Can you work these out from the model? Positions are in its coordinate system, mm. Face numbers are marked on the shaded views. Give positions to 0.01 mm unless a question says otherwise; leave off trailing zeros. Loops run counter-clockwise (first coordinate to the right, second up) from the corner with the lowest first, then second, coordinate; pieces in that order, holes last. Notation, with made-up numbers: (41.25, -31) -> (94.25, -31) arc R16 ccw to (94.25, -6) -> close; hole circle Ø5 at (-11.5, 66.5). An arc over 180 degrees is marked (long way). Return JSON: item names as keys, results as strings. Group by question number.
Q1. Suppose I cut it at B-B, the plane y = -1.9. Please give me the cut outline in (x, z) (3 decimals).
Q2. Thinking about a two-plate mould opening in Y: for the marked faces 1 and 2, which applies, pulls with the +Y half, pulls with the -Y half, needs draft (parallel to the pull), parting line crosses it, or undercut?
Q3. Suppose I cut it at C-C, the plane z = -34. Please give me the cut outline in (x, y).
Q4. Suppose I cut it at A-A, the plane z = -18.35. Please give me the cut outline in (x, y), and give its area (3 significant figures).
Q5. Suppose I cut it at D-D, the plane x = 14.5. Please give me the cut outline in (y, z) (3 decimals), and give its area (3 significant figures).
Q6. I need wall thicknesses on line 1 along X through (y, z) = (-1.85, -18.35); line 2 along X through (y, z) = (-1.05, -44.5); line 3 along X through (y, z) = (-0.75, -6.5). Which ranges of each line are inside material? Lowest first, please. Write a range as [from, to].
Q7. Will these pins go through, and if not, where does the flat tip stop? pin 1 (1.6 mm diameter, centred on x = 2, y = -1, fed in from -Z) (3 decimals); pin 2 (1 mm diameter, centred on y = -3, z = -37, fed in from +X); pin 3 (1.5 mm diameter, centred on x = 13, y = -2.5, fed in from +Z).
```python
from build123d import *

# Parameters (mm, degrees)
BASE_FLANGE1_START        = -3.2
BASE_FLANGE1_DEPTH        = 3.2
SKETCH8_R                 = 1.635
CUT_EXTRUDE1_DEPTH        = 3.2
F_4_CLEARANCE_HOLE1_D     = 3.2639
F_4_CLEARANCE_HOLE1_DEPTH = 3.2
F_4_CLEARANCE_HOLE1_TIP   = 0.980574487
CUT_EXTRUDE2_DEPTH        = 3.2


# Read off the part's stored shape, not the designer's step: Base-Flange1
with BuildPart() as part:
    # Base-Flange1 outline → Base-Flange1 (new body)
    with BuildSketch(Plane(origin=(0, 0, 0), x_dir=(1, 0, 0), z_dir=(0, 1, 0)).offset(BASE_FLANGE1_START)):
        with BuildLine():
            ThreePointArc((-29.358964924, 3.232453337), (-23.15, 7), (-16.941035076, 3.232453337))
            ThreePointArc((-16.941035076, 3.232453337), (-11.575, 1.808851774), (-6.208964924, 3.232453337))
            ThreePointArc((-6.208964924, 3.232453337), (0, 7), (6.208964924, 3.232453337))
            ThreePointArc((6.208964924, 3.232453337), (11.575, 1.808851774), (16.941035076, 3.232453337))
            ThreePointArc((16.941035076, 3.232453337), (23.15, 7), (29.358964924, 3.232453337))
            Line((29.358964924, 3.232453337), (29.358964924, 25.825))
            Line((29.358964924, 25.825), (-19.358964924, 25.825))
            Line((-19.358964924, 25.825), (-19.358964924, 48.325))
            Line((-19.358964924, 48.325), (-29.358964924, 48.325))
            Line((-29.358964924, 48.325), (-29.358964924, 3.232453337))
        make_face()
    extrude(amount=BASE_FLANGE1_DEPTH)

    # Sketch8 → Cut-Extrude1 (cut)
    with BuildSketch(Plane(origin=(0, 0, 0), x_dir=(1, 0, 0), z_dir=(0, 1, 0))):
        with Locations(Location((-24.358964924, 44.325, 0), (0, 0, 270))):
            Circle(SKETCH8_R)
        with Locations(Location((-24.358964924, 34.825, 0), (0, 0, 270))):
            Circle(SKETCH8_R)
    extrude(amount=-CUT_EXTRUDE1_DEPTH, mode=Mode.SUBTRACT)

    # #4 Clearance Hole1
    with Locations(Plane(origin=(0, 0, 0), x_dir=(1, 0, 0), z_dir=(0, 1, 0))):
        with Locations((11.575, 18.35), (-11.575, 18.35)):
            Hole(F_4_CLEARANCE_HOLE1_D / 2, depth=F_4_CLEARANCE_HOLE1_DEPTH)
            with Locations((0, 0, -(F_4_CLEARANCE_HOLE1_DEPTH + F_4_CLEARANCE_HOLE1_TIP / 2))):  # 118° drill point
                Cone(0, F_4_CLEARANCE_HOLE1_D / 2, F_4_CLEARANCE_HOLE1_TIP, mode=Mode.SUBTRACT)

    # Sketch12 → Cut-Extrude2 (cut)
    with BuildSketch(Plane(origin=(0, 0, 0), x_dir=(1, 0, 0), z_dir=(0, 1, 0))):
        with BuildLine():
            Line((-29.802462418, 3.463342862), (-29.802462418, -1.121913875))
            Line((-29.802462418, -1.121913875), (35.30589457, -1.121913875))
            Line((35.30589457, -1.121913875), (35.30589457, 25.825))
            Line((35.30589457, 25.825), (28.858964924, 25.825))
            Line((28.858964924, 25.825), (28.858964924, 4.863920178))
            ThreePointArc((28.858964924, 4.863920178), (22.380832381, 7.460454488), (16.568740084, 3.596806627))
            ThreePointArc((16.568740084, 3.596806627), (11.575, 2.308851774), (6.581259916, 3.596806627))
            ThreePointArc((6.581259916, 3.596806627), (0, 7.5), (-6.581259916, 3.596806627))
            ThreePointArc((-6.581259916, 3.596806627), (-11.575, 2.308851774), (-16.568740084, 3.596806627))
            ThreePointArc((-16.568740084, 3.596806627), (-23.225634604, 7.499618617), (-29.802462418, 3.463342862))
        make_face()
    extrude(amount=-CUT_EXTRUDE2_DEPTH, mode=Mode.SUBTRACT)


solid = part.part
```
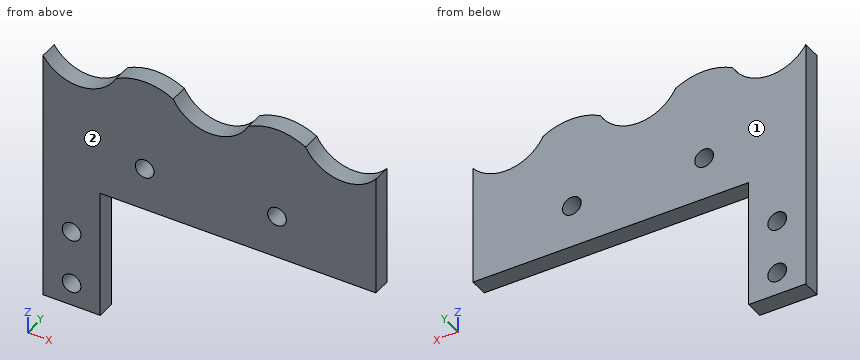
Ans:
{
 "1": {"outline": "(-29.359, -48.325) -> (-19.359, -48.325) -> (-19.359, -25.825) -> (28.859, -25.825) -> (28.859, -4.864) arc R7.5 cw to (16.569, -3.597) arc R10.325 ccw to (6.581, -3.597) arc R7.5 cw to (-6.581, -3.597) arc R10.325 ccw to (-16.569, -3.597) arc R7.5 cw to (-29.359, -4.207) -> close; hole circle Ø3.27 at (-24.359, -44.325); hole circle Ø3.27 at (-24.359, -34.825); hole circle Ø3.264 at (-11.575, -18.35); hole circle Ø3.264 at (11.575, -18.35)"},
 "2": {"face 1": "pulls with the +Y half", "face 2": "pulls with the -Y half"},
 "3": {"outline": "(-29.36, -3.2) -> (-25.77, -3.2) -> (-25.77, 0) -> (-29.36, 0) -> close; (-22.95, -3.2) -> (-19.36, -3.2) -> (-19.36, 0) -> (-22.95, 0) -> close"},
 "4": {"outline": "(-29.36, -3.2) -> (-13.21, -3.2) -> (-13.21, 0) -> (-29.36, 0) -> close; (-9.94, -3.2) -> (9.94, -3.2) -> (9.94, 0) -> (-9.94, 0) -> close; (13.21, -3.2) -> (28.86, -3.2) -> (28.86, 0) -> (13.21, 0) -> close", "area": "165 mm^2"},
 "5": {"outline": "(-3.2, -25.825) -> (0, -25.825) -> (0, -2.732) -> (-3.2, -2.732) -> close", "area": "73.9 mm^2"},
 "6": {"line 1": "x = [-29.36, -13.21], [-9.94, 9.94], [13.21, 28.86]", "line 2": "x = [-29.36, -25.98], [-22.73, -19.36]", "line 3": "x = [-29.36, -26.89], [-19.41, -3.74], [3.74, 19.41], [26.89, 28.86]"},
 "7": {"pin 1": "stops at z = -25.825", "pin 2": "stops at x = -19.36", "pin 3": "stops at z = -2.33"}
}
